```python
from build123d import *

# Parameters (mm, degrees)
PAD_DEPTH       = 74
PAD001_DEPTH    = 17
PAD002_DEPTH    = 49
PAD003_DEPTH    = 35
PAD004_DEPTH    = 17
PAD005_DEPTH    = 39
PAD006_DEPTH    = 18
PAD007_DEPTH    = 17
PAD008_DEPTH    = 24
POCKET_DEPTH    = 74
POCKET001_DEPTH = 17
POCKET002_DEPTH = 49
POCKET003_DEPTH = 37
POCKET004_DEPTH = 17
POCKET005_DEPTH = 42
POCKET006_DEPTH = 20
POCKET007_DEPTH = 17
POCKET008_DEPTH = 24
SKETCH020_W     = 3
SKETCH020_H     = 5
PAD009_DEPTH    = 75
SKETCH021_W     = 2
SKETCH021_H     = 3
POCKET009_DEPTH = 75
POCKET010_DEPTH = 2
SKETCH023_W     = 3
SKETCH023_H     = 5
PAD010_DEPTH    = 75
SKETCH024_W     = 2
SKETCH024_H     = 3
POCKET011_DEPTH = 75
POCKET012_DEPTH = 3


with BuildPart() as part:
    # Sketch → Pad (new body)
    with BuildSketch(Plane.XY):
        Polygon((0, 0), (15, 0), (15, -2), (14, -3), (1, -3), (0, -2), align=None)
    extrude(amount=PAD_DEPTH)

    # Sketch002 (on Face8 of Pad) → Pad001 (join)
    with BuildSketch(Plane.XY.offset(74)):
        Polygon((-2, 0), (13, 0), (13, -2), (12, -3), (-1, -3), (-2, -2), align=None)
    extrude(amount=PAD001_DEPTH)

    # Sketch003 (on Face13 of Pad001) → Pad002 (join)
    with BuildSketch(Plane.XY.offset(91)):
        Polygon((1, 0), (16, 0), (16, -2), (15, -3), (2, -3), (1, -2), align=None)
    extrude(amount=PAD002_DEPTH)

    # Sketch004 (on Face21 of Pad002) → Pad003 (join)
    with BuildSketch(Plane(origin=(15, 0, 0), x_dir=(0, 0, -1), z_dir=(1, 0, 0))):
        Polygon((-113, 0), (-98, 0), (-98, -2), (-99, -3), (-112, -3), (-113, -2), align=None)
    extrude(amount=PAD003_DEPTH)

    # Sketch005 (on Face33 of Pad003) → Pad004 (join)
    with BuildSketch(Plane(origin=(50, 0, 0), x_dir=(0, 0, -1), z_dir=(1, 0, 0))):
        Polygon((-107, 0), (-92, 0), (-92, -2), (-93, -3), (-106, -3), (-107, -2), align=None)
    extrude(amount=PAD004_DEPTH)

    # Sketch006 (on Face38 of Pad004) → Pad005 (join)
    with BuildSketch(Plane(origin=(0, 0, 93), x_dir=(-1, 0, 0), z_dir=(0, 0, -1))):
        Polygon((-73, 0), (-58, 0), (-58, -2), (-59, -3), (-72, -3), (-73, -2), align=None)
    extrude(amount=PAD005_DEPTH)

    # Sketch007 (on Face45 of Pad005) → Pad006 (join)
    with BuildSketch(Plane.ZY.offset(-59)):
        Polygon((44, 0), (59, 0), (59, -2), (58, -3), (45, -3), (44, -2), align=None)
    extrude(amount=PAD006_DEPTH)

    # Sketch008 (on Face58 of Pad006) → Pad007 (join)
    with BuildSketch(Plane.ZY.offset(-41)):
        Polygon((42, 0), (57, 0), (57, -2), (56, -3), (43, -3), (42, -2), align=None)
    extrude(amount=PAD007_DEPTH)

    # Sketch009 (on Face66 of Pad007) → Pad008 (join)
    with BuildSketch(Plane.ZY.offset(-24)):
        Polygon((44, 0), (59, 0), (59, -2), (58, -3), (45, -3), (44, -2), align=None)
    extrude(amount=PAD008_DEPTH)

    # Sketch010 (on Face2 of Pad008) → Pocket (cut)
    with BuildSketch(Plane(origin=(0, 0, 0), x_dir=(1, 0, 0), z_dir=(0, 0, -1))):
        Polygon((2.5, 2), (12.5, 2), (12.5, 1.5), (12, 1.5), (12, 0), (3, 0), (3, 1.5), (2.5, 1.5), align=None)
    extrude(amount=-POCKET_DEPTH, mode=Mode.SUBTRACT)

    # Sketch012 (on Face38 of Pocket) → Pocket001 (cut)
    with BuildSketch(Plane(origin=(0, 0, 74), x_dir=(1, 0, 0), z_dir=(0, 0, -1))):
        Polygon((0.5, 2), (10.5, 2), (10.5, 1.5), (10, 1.5), (10, 0), (1, 0), (1, 1.5), (0.5, 1.5), align=None)
    extrude(amount=-POCKET001_DEPTH, mode=Mode.SUBTRACT)

    # Sketch013 (on Face68 of Pocket001) → Pocket002 (cut)
    with BuildSketch(Plane(origin=(0, 0, 91), x_dir=(1, 0, 0), z_dir=(0, 0, -1))):
        Polygon((3.5, 2), (13.5, 2), (13.5, 1.5), (13, 1.5), (13, 0), (4, 0), (4, 1.5), (3.5, 1.5), align=None)
    extrude(amount=-POCKET002_DEPTH, mode=Mode.SUBTRACT)

    # Sketch014 (on Face102 of Pocket002) → Pocket003 (cut)
    with BuildSketch(Plane(origin=(50, 0, 0), x_dir=(0, 0, 1), z_dir=(1, 0, 0))):
        Polygon((100.5, 2), (110.5, 2), (110.5, 1.5), (110, 1.5), (110, 0), (101, 0), (101, 1.5), (100.5, 1.5), align=None)
    extrude(amount=-POCKET003_DEPTH, mode=Mode.SUBTRACT)

    # Sketch015 (on Face132 of Pocket003) → Pocket004 (cut)
    with BuildSketch(Plane(origin=(67, 0, 0), x_dir=(0, 0, 1), z_dir=(1, 0, 0))):
        Polygon((94.5, 2), (104.5, 2), (104.5, 1.5), (104, 1.5), (104, 0), (95, 0), (95, 1.5), (94.5, 1.5), align=None)
    extrude(amount=-POCKET004_DEPTH, mode=Mode.SUBTRACT)

    # Sketch016 (on Face132 of Pocket004) → Pocket005 (cut)
    with BuildSketch(Plane(origin=(0, 0, 54), x_dir=(1, 0, 0), z_dir=(0, 0, -1))):
        Polygon((60.5, 2), (70.5, 2), (70.5, 1.5), (70, 1.5), (70, 0), (61, 0), (61, 1.5), (60.5, 1.5), align=None)
    extrude(amount=-POCKET005_DEPTH, mode=Mode.SUBTRACT)

    # Sketch017 (on Face115 of Pocket005) → Pocket006 (cut)
    with BuildSketch(Plane(origin=(61, 0, 0), x_dir=(0, 0, 1), z_dir=(1, 0, 0))):
        Polygon((46.5, 2), (56.5, 2), (56.5, 1.5), (56, 1.5), (56, 0), (47, 0), (47, 1.5), (46.5, 1.5), align=None)
    extrude(amount=-POCKET006_DEPTH, mode=Mode.SUBTRACT)

    # Sketch018 (on Face90 of Pocket006) → Pocket007 (cut)
    with BuildSketch(Plane(origin=(41, 0, 0), x_dir=(0, 0, 1), z_dir=(1, 0, 0))):
        Polygon((44.5, 2), (54.5, 2), (54.5, 1.5), (54, 1.5), (54, 0), (45, 0), (45, 1.5), (44.5, 1.5), align=None)
    extrude(amount=-POCKET007_DEPTH, mode=Mode.SUBTRACT)

    # Sketch019 (on Face19 of Pocket007) → Pocket008 (cut)
    with BuildSketch(Plane(origin=(0, 0, 0), x_dir=(0, 0, -1), z_dir=(-1, 0, 0))):
        Polygon((-56.5, 2), (-46.5, 2), (-46.5, 1.5), (-47, 1.5), (-47, 0), (-56, 0), (-56, 1.5), (-56.5, 1.5), align=None)
    extrude(amount=-POCKET008_DEPTH, mode=Mode.SUBTRACT)

    # Sketch020 (on Face13 of Pocket008) → Pad009 (join)
    with BuildSketch(Plane.YZ.offset(-2)):
        with Locations((-1.5, 2.5)):
            Rectangle(SKETCH020_W, SKETCH020_H)
    extrude(amount=PAD009_DEPTH)

    # Sketch021 (on Face20 of Pad009) → Pocket009 (cut)
    with BuildSketch(Plane.YZ.offset(73)):
        with Locations((-1, 1.5)):
            Rectangle(SKETCH021_W, SKETCH021_H)
    extrude(amount=-POCKET009_DEPTH, mode=Mode.SUBTRACT)

    # Sketch022 (on Face2 of Pocket009) → Pocket010 (cut)
    with BuildSketch(Plane(origin=(0, 0, 3), x_dir=(1, 0, 0), z_dir=(0, 0, -1))):
        Polygon((2.5, 2), (12.5, 2), (12.5, 1.5), (12, 1.5), (12, 0), (3, 0), (3, 1.5), (2.5, 1.5), align=None)
    extrude(amount=-POCKET010_DEPTH, mode=Mode.SUBTRACT)

    # Sketch023 (on Face185 of Pocket010) → Pad010 (join)
    with BuildSketch(Plane.YZ.offset(-1)):
        with Locations((-1.5, 137.5)):
            Rectangle(SKETCH023_W, SKETCH023_H)
    extrude(amount=PAD010_DEPTH)

    # Sketch024 (on Face226 of Pad010) → Pocket011 (cut)
    with BuildSketch(Plane.YZ.offset(74)):
        with Locations((-1, 138.5)):
            Rectangle(SKETCH024_W, SKETCH024_H)
    extrude(amount=-POCKET011_DEPTH, mode=Mode.SUBTRACT)

    # Sketch025 (on Face209 of Pocket011) → Pocket012 (cut)
    with BuildSketch(Plane(origin=(0, 0, 137), x_dir=(-1, 0, 0), z_dir=(0, 0, 1))):
        Polygon((-13.5, 2), (-3.5, 2), (-3.5, 1.5), (-4, 1.5), (-4, 0), (-13, 0), (-13, 1.5), (-13.5, 1.5), align=None)
    extrude(amount=-POCKET012_DEPTH, mode=Mode.SUBTRACT)


solid = part.part
```
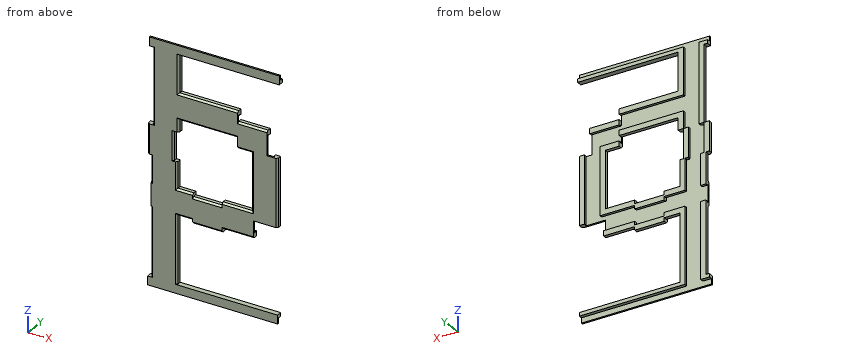
The listing builds one solid part. Answer for the finished solid, in the listing's coordinates (mm). Coordinates: 2 decimals unless noted, no trailing zeros. Loops run counter-clockwise (first coordinate to the right, second up) from the corner with the lowest first, then second, coordinate; pieces in that order, holes last. Notation, with made-up numbers: M -12,-24.5 L 1,-24.5 A27 ccw 1,7.5 Z; hole C 75,17 d1. An arc over 180 degrees is marked long. Answer as CSV lines item,"result". Start each with the question number.
(1) The part is cut by section B-B (z = 122). Give the vertices of the cut face in (x, y).
(2) Find the intervals of material crossed by L1, parallel to Z at x = 55, y = -0.7; L2, parallel to Z at x = 23, y = -0.25; L3, parallel to X at y = -1.75, z = 61.5, in increasing order. Write a range as [from, to].
(3) The part is cut by section D-D (x = 8.5). Give the vertices of the cut face in (y, z).
(4) The part is cut by section C-C (x = 48). State how many separate pieces and enclosed holes the cut face has, and give its area (3 significant figures).
(5) The part is cut by section A-A (z = 78). Give the vertices of the cut face in (x, y), and give its area (3 significant figures).
(6) Given pin 1 (1 mm diameter, centred on x = 12, y = -0.5, fed in from -Z); pin 2 (1.6 mm diameter, centred on y = -0.5, z = 97.5, fed in from -X); pin 3 (1.5 mm diameter, centred on y = -0.5, z = 45.5, fed in from +X), each flat-ended and moving along its own axis, determine where each tip first touches the part or whether it passes through.
Determined:
1,outline,"M 1,-2 L 2,-3 L 15,-3 L 16,-2 L 16,0 L 13,0 L 13,-1.5 L 13.5,-1.5 L 13.5,-2 L 3.5,-2 L 3.5,-1.5 L 4,-1.5 L 4,0 L 1,0 Z"
2,L1,"[3, 5], [44, 47], [56, 59], [92, 95], [104, 107], [135, 137]"
2,L2,"[3, 5], [44, 47], [56, 59], [98, 101], [110, 113], [135, 137]"
2,L3,"[0, 2.5], [12.5, 15], [58, 60.5], [70.5, 73]"
3,outline,"M -3,0 L -2,0 L -2,140 L -3,140 Z"
4,separate pieces,"4"
4,enclosed holes,"0"
4,area,"69.0 mm2"
5,outline,"M -2,-2 L -1,-3 L 12,-3 L 13,-2 L 13,0 L 10,0 L 10,-1.5 L 10.5,-1.5 L 10.5,-2 L 0.5,-2 L 0.5,-1.5 L 1,-1.5 L 1,0 L -2,0 Z; M 58,-2 L 59,-3 L 72,-3 L 73,-2 L 73,0 L 70,0 L 70,-1.5 L 70.5,-1.5 L 70.5,-2 L 60.5,-2 L 60.5,-1.5 L 61,-1.5 L 61,0 L 58,0 Z"
5,area,"51.0 mm2"
6,pin 1,"z = 3"
6,pin 2,"x = 1"
6,pin 3,"x = 59"
